For this review, use the dimensioned drawing (mm, ordinates from the lowest corner) and the shaded views. Round coordinates to 2 decimals unless told otherwise and drop trailing zeros. Write each loop counter-clockwise with the first axis right and the second up, starting at its lowest first coordinate (ties: lowest second). Pieces come first, ordered by that corner, then holes.
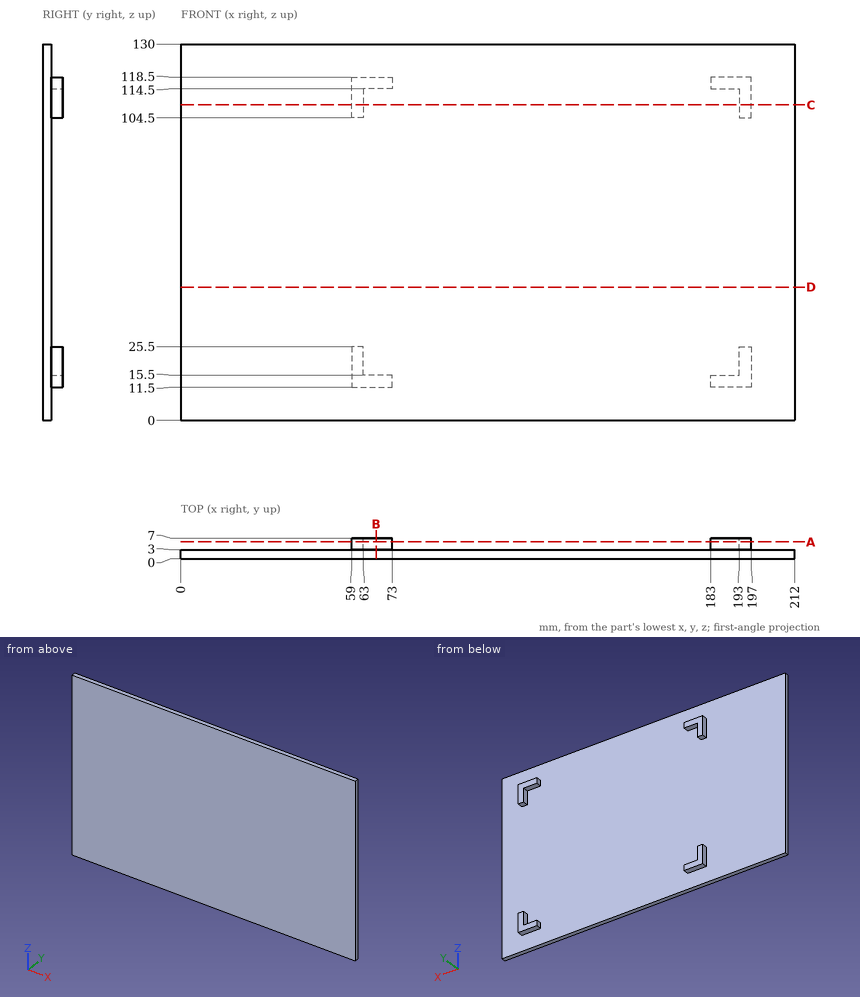
(1) We need section B-B, the plane x = 67.5. Give the boundary of the cut face in (y, z).
Geometry check:
outline: (0, 0) - (3, 0) - (3, 11.5) - (7, 11.5) - (7, 15.5) - (3, 15.5) - (3, 114.5) - (7, 114.5) - (7, 118.5) - (3, 118.5) - (3, 130) - (0, 130) - close
(2) We need section C-C, the plane z = 109. Give the boundary of the cut face in (x, y), and give its area (3 significant figures).
Geometry check:
outline: (0, 0) - (212, 0) - (212, 3) - (197, 3) - (197, 7) - (193, 7) - (193, 3) - (63, 3) - (63, 7) - (59, 7) - (59, 3) - (0, 3) - close
area: 668 mm2
(3) For pin 1 Ø4 at (x, z) = (105.5, 94) entering from -Y; pin 2 Ø3 at (y, z) = (5, 16) entering from +X; pin 3 Ø2 at (x, y) = (189, 5) entering from +Z; pin 4 Ø2 at (y, z) = (5.5, 20) entering from -X, all flat-tipped, find the tip position at first contact; note any pin that passes through.
Geometry check:
pin 1: stops at y = 0
pin 2: stops at x = 197
pin 3: stops at z = 118.5
pin 4: stops at x = 59
(4) We need section A-A, the plane y = 5.75. Give the boundary of the cut face in (x, z), and give its area (3 significant figures).
Geometry check:
outline: (59, 11.5) - (73, 11.5) - (73, 15.5) - (63, 15.5) - (63, 25.5) - (59, 25.5) - close; (59, 104.5) - (63, 104.5) - (63, 114.5) - (73, 114.5) - (73, 118.5) - (59, 118.5) - close; (183, 11.5) - (197, 11.5) - (197, 25.5) - (193, 25.5) - (193, 15.5) - (183, 15.5) - close; (183, 114.5) - (193, 114.5) - (193, 104.5) - (197, 104.5) - (197, 118.5) - (183, 118.5) - close
area: 384 mm2
(5) We need section D-D, the plane z = 46. Give the boundary of the cut face in (x, y).
Geometry check:
outline: (0, 0) - (212, 0) - (212, 3) - (0, 3) - close
(6) For line 1 along X through (y, z) = (3.5, 13.5); line 2 along X through (y, z) = (5, 20); line 3 along Y through (x, z) = (159.5, 13), list the stretches that pass through material, from the lowest coordinate up.
Geometry check:
line 1: x = 59 to 73, 183 to 197
line 2: x = 59 to 63, 193 to 197
line 3: y = 0 to 3
